The listing builds one solid part. Answer for the finished solid, in the listing's coordinates (mm). Give positions to 0.01 mm unless a question says otherwise; leave off trailing zeros. Order: outer loops, then holes, each group sorted by start corner. A loop starts at its lowest first (then second) coordinate and runs counter-clockwise, first axis right, second up.
```python
from build123d import *

# Parameters (mm, degrees)
SKETCH4_R               = 6.75
SKETCH4_R_2             = 4.75
BOSS_EXTRUDE4_DEPTH     = 15
FILLET3_R               = 2
FILLET4_R               = 2
CUT_EXTRUDE1_DEPTH      = 16.333786269
CUT_EXTRUDE1_DEPTH_BACK = 16.333786269


with BuildPart() as part:
    # Sketch4 → Boss-Extrude4 (new body)
    with BuildSketch(Plane.ZY.offset(-12)):
        with Locations(Location((0, 0, 0), (0, 0, 270))):
            Circle(SKETCH4_R)
        with Locations(Location((0, 0, 0), (0, 0, 270))):
            Circle(SKETCH4_R_2, mode=Mode.SUBTRACT)
    extrude(amount=BOSS_EXTRUDE4_DEPTH)

    # Fillet3
    fillet3_edges = [part.edges().sort_by_distance(p)[0] for p in [
        (12, 6.75, 0),
    ]]
    fillet(fillet3_edges, radius=FILLET3_R - 0.0001)  # a hair under: the kernel refuses the full size

    # Fillet4
    fillet4_edges = [part.edges().sort_by_distance(p)[0] for p in [
        (-3, 6.75, 0),
    ]]
    fillet(fillet4_edges, radius=FILLET4_R - 0.0001)  # a hair under: the kernel refuses the full size

    # Sketch5 → Cut-Extrude1 (cut, two sides: drawn at the far end of the back side and taken through both)
    with BuildSketch(Plane(origin=(0, 0, 0), x_dir=(0, 0, -1), z_dir=(1, 0, 0)).offset(-CUT_EXTRUDE1_DEPTH_BACK)):
        with BuildLine():
            ThreePointArc((6.75, 0), (0, 6.75), (-6.75, 0))
            Line((-6.75, 0), (-4.75, 0))
            ThreePointArc((-4.75, 0), (0, 4.75), (4.75, 0))
            Line((4.75, 0), (6.75, 0))
        make_face()
    extrude(amount=CUT_EXTRUDE1_DEPTH + CUT_EXTRUDE1_DEPTH_BACK, mode=Mode.SUBTRACT)


solid = part.part
```
1) Find section A-A (x = 1). Write down the section's boundary in (y, z), then the cut area to 3 significant figures.
Geometry says:
outline: (0, -6.75) - (0, -4.75) arc R4.75 cw to (0, 4.75) - (0, 6.75) arc R6.75 ccw to start
area: 36.1 mm2
2) Given P1, Ø2, axis at x = 0, y = -3, coming from the -Z side, flat-ended and moving along its own axis, determine where the tip first touches the part or whether it passes through.
Geometry says:
P1: stops at z = -6.45
3) Straight lines are drawn through the part: probe 1 along Z at (x, y) = (10.5, -0.5); probe 2 along Z at (x, y) = (0.75, -2.5); probe 3 along Y at (x, z) = (4.5, 1). For each, find the intervals that lie inside material, in ascending order.
Geometry says:
probe 1: z = -6.67 to -4.72, 4.72 to 6.67
probe 2: z = -6.27 to -4.04, 4.04 to 6.27
probe 3: y = -6.68 to -4.64
4) For a pull along Z with two mould halves and no side action, classify faces 1 (the flat face through (4, 0, 6)), 2 (the cylindrical face through (4.61, -4.75, -0.1)), 3 (the cylindrical face through (4.58, -6.75, -0.15)) as +Z half, -Z half, draft (parallel to the pull), parting line (faces both ways), or undercut.
Geometry says:
face 1: draft
face 2: undercut
face 3: parting line
